The model under review builds one solid part; all positions refer to its coordinate system, in mm. Face numbers are marked on the shaded views. Round coordinates to 2 decimals unless told otherwise and drop trailing zeros. Loops run counter-clockwise (first coordinate to the right, second up) from the corner with the lowest first, then second, coordinate; pieces in that order, holes last. Notation, with made-up numbers: M -9,8 L 12,8 A18 ccw 12,25 Z; hole C -4.5,-27 d3. An arc over 180 degrees is marked long. Answer as a JSON object with one key per item and string values. Group by question number.
Item 1: Consider section C-C (z = -8). Give the boundary of the cut face in (x, y), and give its area (3 significant figures).
Item 2: Insertion check: P1, Ø5.5, axis at x = -9.8, y = 33.8, coming from the -Z side. The pin has a flat end and moves straight along its axis. Give the tip position at first contact, or say it passes through.
Item 3: The part is to be moulded in two halves that separate along X. For the marked faces 1, 2 and 3, say which applies: +X half, -X half, draft (parallel to the pull), parting line (faces both ways), or undercut.
Item 4: To check wall thickness, follow line 1 (Y direction, x = -9.8, z = -4.25); line 2 (X direction, y = 8, z = -9.5); line 3 (X direction, y = 34, z = -6). State the ranges of each line that lie inside material, in increasing order.
Item 5: Consider section B-B (y = 33.8). Give the boundary of the cut face in (x, z), and give its area (3 significant figures).
Item 6: Consider section D-D (z = -2.75). Give the boundary of the cut face in (x, y), and give its area (3 significant figures).
Item 7: Consider section A-A (x = 9.8). Give the boundary of the cut face in (y, z), and give its area (3 significant figures).
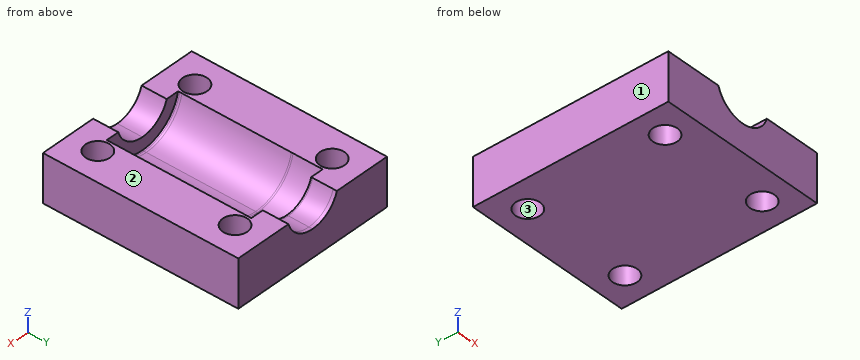
Solid Edge part; units mm, degrees
sketch "Sketch1" plane through (0, 0, 0) normal (0, 0, 1) x (1, 0, 0)
  circle A0 centre (-9.8, 33.8) radius 2.2
  circle A1 centre (-9.8, 9.2) radius 2.2
  circle A2 centre (9.8, 9.2) radius 2.2
  circle A3 centre (9.8, 33.8) radius 2.2
  line L0 (-15, 4) -> (15, 4)
  line L1 (15, 4) -> (15, 39)
  line L2 (15, 39) -> (-15, 39)
  line L3 (-15, 39) -> (-15, 4)
  dimension "D1" = 15
  dimension "D2" = 15
  dimension "D3" = 9.8
extrude "Protrusion1" add sketch "Sketch1" against normal blind 10
sketch "Sketch2" plane through (0, 0, 0) normal (1, 0, 0) x (0, 1, 0)
  line L0 (8.8, -7.35) -> (8.5, -7.35)
  line L1 (8.5, -7.35) -> (8.5, -5.1123)
  line L2 (2.721, -5.1123) -> (8.5, -5.1123)
  line L3 (2.721, -5.1123) -> (-1.0103, -5.1123)
  line L4 (-1.0103, -5.1123) -> (-1.0103, -3.9681)
  line L5 (-1.0103, -2.774) -> (-1.0103, -3.9681)
  line L6 (-12.5526, -2.774) -> (-1.0103, -2.774)
  line L7 (-12.5526, 0) -> (-12.5526, -2.774)
  line L8 (39.4373, 0) -> (-12.5526, 0)
  line L9 (39.4373, -5.1123) -> (39.4373, 0)
  line L10 (38.3428, -5.1123) -> (39.4373, -5.1123)
  line L11 (34.6612, -5.1123) -> (38.3428, -5.1123)
  line L12 (34.4, -5.1123) -> (34.6612, -5.1123)
  line L13 (34.4, -7.3511) -> (34.4, -5.1123)
  line L14 (29.1, -7.3511) -> (34.4, -7.3511)
  line L15 (29.1, -7.3511) -> (28.8, -7.3511)
  line L16 (9.2, -7.35) -> (28.8, -7.3511)
  line L17 (8.8023, -7.35) -> (9.2, -7.35)
  dimension "D1" = 8.8
  dimension "D2" = 8.5
revolve "RevolvedCutout1" cut sketch "Sketch2" angle 360 about axis through (0, -60, 0) along (0, 1, 0)
sketch "Sketch3" plane through (0, 4, -5) normal (0, -1, 0) x (1, 0, 0)
  line L0 (-23.1839, 5) -> (21.8988, 5)
  line L1 (21.8988, 5) -> (21.8988, 3.5)
  line L2 (21.8988, 3.5) -> (-23.1839, 3.5)
  line L3 (-23.1839, 3.5) -> (-23.1839, 5)
  dimension "D1" = 23.1839
extrude "ExtrudedCutout_2" cut sketch "Sketch3" against normal blind 318.8634
Geometry results:
{
 "1": {"outline": "M -15,4 L 15,4 L 15,39 L -15,39 Z; hole C -9.8,9.2 d4.4; hole C -9.8,33.8 d4.4; hole C 9.8,9.2 d4.4; hole C 9.8,33.8 d4.4", "area": "989 mm^2"},
 "2": {"P1": "stops at z = -10"},
 "3": {"face 1": "-X half", "face 2": "draft", "face 3": "undercut"},
 "4": {"line 1": "y = 4 to 7, 11.4 to 31.6, 36 to 39", "line 2": "x = -15 to -11.64, -7.96 to 7.96, 11.64 to 15", "line 3": "x = -15 to -11.99, -7.61 to -4.25, 4.25 to 7.61, 11.99 to 15"},
 "5": {"outline": "M -15,-10 L -12,-10 L -12,-1.5 L -15,-1.5 Z; M -7.6,-10 L 7.6,-10 L 7.6,-1.5 L 7.2,-1.5 A7.35 cw -7.2,-1.5 L -7.6,-1.5 Z; M 12,-10 L 15,-10 L 15,-1.5 L 12,-1.5 Z", "area": "117 mm^2"},
 "6": {"outline": "M -15,4 L -4.31,4 L -4.31,8.5 L -6.82,8.5 L -6.82,28.8 L -6.82,34.4 L -4.31,34.4 L -4.31,39 L -15,39 Z; M 4.31,4 L 15,4 L 15,39 L 4.31,39 L 4.31,34.4 L 6.82,34.4 L 6.82,28.8 L 6.82,8.5 L 4.31,8.5 Z; hole C -9.8,9.2 d4.4; hole C -9.8,33.8 d4.4; hole C 9.8,9.2 d4.4; hole C 9.8,33.8 d4.4", "area": "558 mm^2"},
 "7": {"outline": "M 4,-10 L 7,-10 L 7,-1.5 L 4,-1.5 Z; M 11.4,-10 L 31.6,-10 L 31.6,-1.5 L 11.4,-1.5 Z; M 36,-10 L 39,-10 L 39,-1.5 L 36,-1.5 Z", "area": "223 mm^2"}
}
